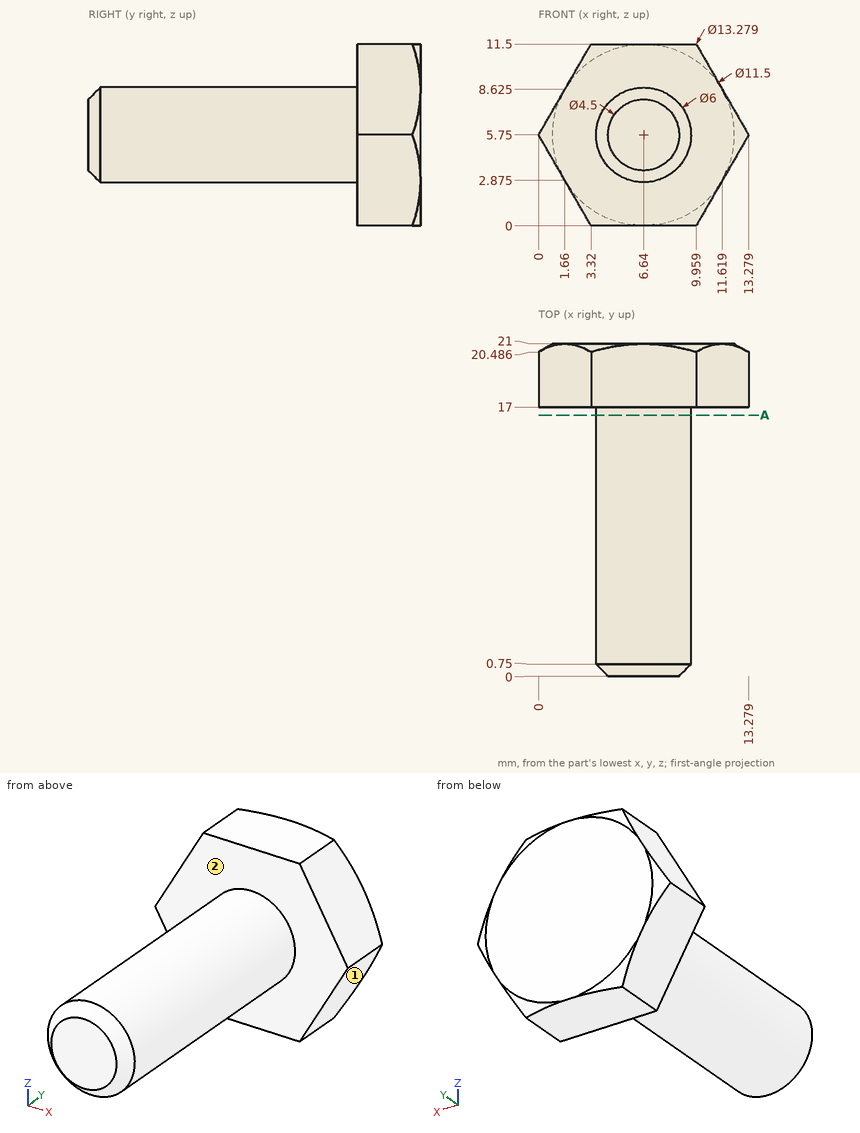
Study the drawing (mm; zero at the part's minimum x, y, z) and answer. A direction names the side the tool comes from. Coordinates: 2 decimals unless noted, no trailing zeros. Write each loop counter-clockwise with the first axis right and the second up, starting at its lowest first coordinate (ties: lowest second). Pieces come first, ordered by that corner, then holes. Notation, with made-up numbers: (82, -10.75) -> (86, -10.75) arc R25 cw to (86, 10.25) -> close; hole circle Ø10 at (68, -18). An arc over 180 degrees is marked (long way). Write item = value, one per line.
(1) Given pin 1 Ø6 at (x, y) = (11, 11.5) entering from +Z (1 decimal); pin 2 Ø5 at (y, z) = (12.5, 3) entering from -X; pin 3 Ø1.5 at (x, z) = (5.5, 9.5) entering from -Y, each flat-ended and moving along its own axis, determine where each tip first touches the part or whether it passes through.
From the geometry:
pin_1 = 8.4
pin_2 = 3.65
pin_3 = 17
(2) Section A-A on y = 16.5 is taken. Write down the section's boundary in (x, z), plus the area to 3 significant figures.
From the geometry:
outline = circle Ø6 at (6.64, 5.75)
area = 28.3 mm2
(3) Straight lines are drawn through the part: L1, parallel to Y at x = 3.75, z = 1; L2, parallel to X at y = 19, z = 4.75; L3, parallel to X at y = 13.75, z = 3.25 (1 decimal). For each, find the intervals that lie inside material, in ascending order. Write a range as from..to.
From the geometry:
L1 = 17..21
L2 = 0.58..12.7
L3 = 5..8.3
(4) Which of the six approach directions +Z, -Z, +X, -X, +Y, -Y give full straight-line access (tool end or side, diameter ignored) to the marked faces 1 and 2?
From the geometry:
face_1 = -Z, +X, +Y, -Y
face_2 = -Y
